```python
from build123d import *

# Parameters (mm, degrees)
KUGGLUCKA_DEPTH  = 12.8
CIRPATTERN_COUNT = 28
RITNING_4_R      = 3
AXELH_L_DEPTH    = 35.443940323


with BuildPart() as part:
    # Ritning 1 → Kugghjulsämne (revolve)
    with BuildSketch(Plane(origin=(0, 0, 0), x_dir=(0, 0, -1), z_dir=(1, 0, 0)), mode=Mode.PRIVATE) as kugghjuls_mne_sk:
        Polygon((6.4, 6.495), (6.4, 2.505), (14.2, 2.505), (14.2, -6.495), (6.4, -6.495), (-6.4, -6.495), (-6.4, 6.495), align=None)
    revolve(kugghjuls_mne_sk.sketch.rotate(Axis((0, -6.495, 6.4), (0, 0, -1)), 90), axis=Axis((0, -6.495, 6.4), (0, 0, -1)))

    # Ritning 2 → Kugglucka (cut)
    with BuildSketch(Plane.XY.offset(6.4)):
        with BuildLine():
            Line((1.302513782, 6.429533177), (1.302513782, 7.549533177))
            Line((1.302513782, 7.549533177), (-1.302513782, 7.549533177))
            Line((-1.302513782, 7.549533177), (-1.302513782, 6.429533177))
            ThreePointArc((-1.302513782, 6.429533177), (-1.099900528, 6.373277677), (-0.988661303, 6.194832596))
            ThreePointArc((-0.988661303, 6.194832596), (0, 5.375), (0.988661303, 6.194832596))
            ThreePointArc((0.988661303, 6.194832596), (1.099900528, 6.373277677), (1.302513782, 6.429533177))
        make_face()
    kugglucka = extrude(amount=-KUGGLUCKA_DEPTH, mode=Mode.SUBTRACT)

    # CirPattern: Kugglucka ×28 about axis
    cirpattern_axis = Axis((0, -6.495, 0), (0, 0, 1))
    for i in range(1, CIRPATTERN_COUNT):
        add(kugglucka.rotate(cirpattern_axis, i * 360 / CIRPATTERN_COUNT), mode=Mode.SUBTRACT)

    # Ritning 3 → Flänsar (revolve)
    with BuildSketch(Plane(origin=(0, 0, 0), x_dir=(0, 0, -1), z_dir=(1, 0, 0))):
        Polygon((-5.9, 4.7815), (-6.4, 4.7815), (-6.4, 6.495), (-7.170628684, 9.371025404), (-6.670628684, 9.505), (-5.9, 6.628974596), align=None)
        Polygon((5.9, 4.7815), (6.4, 4.7815), (6.4, 6.495), (7.170628684, 9.371025404), (6.670628684, 9.505), (5.9, 6.628974596), align=None)
    revolve(axis=Axis((0, -6.495, -6.4), (0, 0, 1)))

    # Ritning 4 → Axelhål (cut, through all)
    with BuildSketch(Plane.XY.offset(6.4)):
        with Locations((0, -6.495)):
            Circle(RITNING_4_R)
    extrude(amount=-AXELH_L_DEPTH, mode=Mode.SUBTRACT)


solid = part.part
```
Verification items for the finished model (mm, model axes). A direction names the side the tool comes from. Round coordinates to 2 decimals unless told otherwise and drop trailing zeros. Order: outer loops, then holes, each group sorted by start corner. A loop starts at its lowest first (then second) coordinate and runs counter-clockwise, first axis right, second up.
1) Material ranges on line 1 (Y direction, x = 0, z = -1) (3 decimals); line 2 (Y direction, x = 0, z = -9.25) (3 decimals); line 3 (X direction, y = 4.5, z = -0.25), recorded low to high.
Geometry says:
line 1: y = -18.365 to -9.495, -3.495 to 5.375
line 2: y = -15.495 to -9.495, -3.495 to 2.505
line 3: x = -6.92 to -6.39, -4.78 to 4.78, 6.39 to 6.92
2) Depth check by flat-ended pin: pin 1 (8 mm diameter, centred on x = 5, y = -15.5, fed in from +Z); pin 2 (1.5 mm diameter, centred on x = 11, y = -9, fed in from -Z); pin 3 (12 mm diameter, centred on x = 11, z = -4, fed in from +Y); pin 4 (2 mm diameter, centred on x = 2, y = -8, fed in from -Z). Enter the tip coordinate at first touch or a pass-through.
Geometry says:
pin 1: stops at z = 6.75
pin 2: stops at z = -6.4
pin 3: stops at y = 8.48
pin 4: stops at z = -14.2
3) Draft check along Z on faces 4 (the conical face through (8.01, -16.95, -6.45)), 5 (the conical face through (8.01, -16.95, 6.45)), 6 (the cylindrical face through (7.42, -15.76, 0.08)). Enter one of: +Z half, -Z half, draft (parallel to the pull), parting line (faces both ways), or undercut.
Geometry says:
face 4: -Z half
face 5: +Z half
face 6: undercut
4) Cross-section at A-A, the plane x = 0. Record the cut outline in (y, z) (3 decimals), plus the area to 3 significant figures.
Geometry says:
outline: (-22.495, -6.671) - (-22.361, -7.171) - (-19.485, -6.4) - (-15.495, -6.4) - (-15.495, -14.2) - (-9.495, -14.2) - (-9.495, 6.4) - (-19.485, 6.4) - (-22.361, 7.171) - (-22.495, 6.671) - (-19.619, 5.9) - (-18.365, 5.9) - (-18.365, -5.9) - (-19.619, -5.9) - close; (-3.495, -14.2) - (2.505, -14.2) - (2.505, -6.4) - (6.495, -6.4) - (9.371, -7.171) - (9.505, -6.671) - (6.629, -5.9) - (5.375, -5.9) - (5.375, 5.9) - (6.629, 5.9) - (9.505, 6.671) - (9.371, 7.171) - (6.495, 6.4) - (-3.495, 6.4) - close
area: 329 mm2
5) Cross-section at B-B, the plane z = -9.25. Record the cut outline in (x, y) (3 decimals), plus the area to 3 significant figures.
Geometry says:
outline: circle Ø18 at (0, -6.495); hole circle Ø6 at (0, -6.495)
area: 226 mm2
6) Tool access check on faces 1 (the cylindrical face through (-0.02, 5.375, 0.083)), 2 (the cylindrical face through (9.27, 0.92, 0.08)), 3 (the cylindrical face through (-11.87, -6.51, 0.08)). Record the directions out of +Z, -Z, +X, -X, +Y, -Y that give a thin tool (end or side, any length) a straight path to the whole face; none if there is none.
Geometry says:
face 1: +Y
face 2: none
face 3: -X
